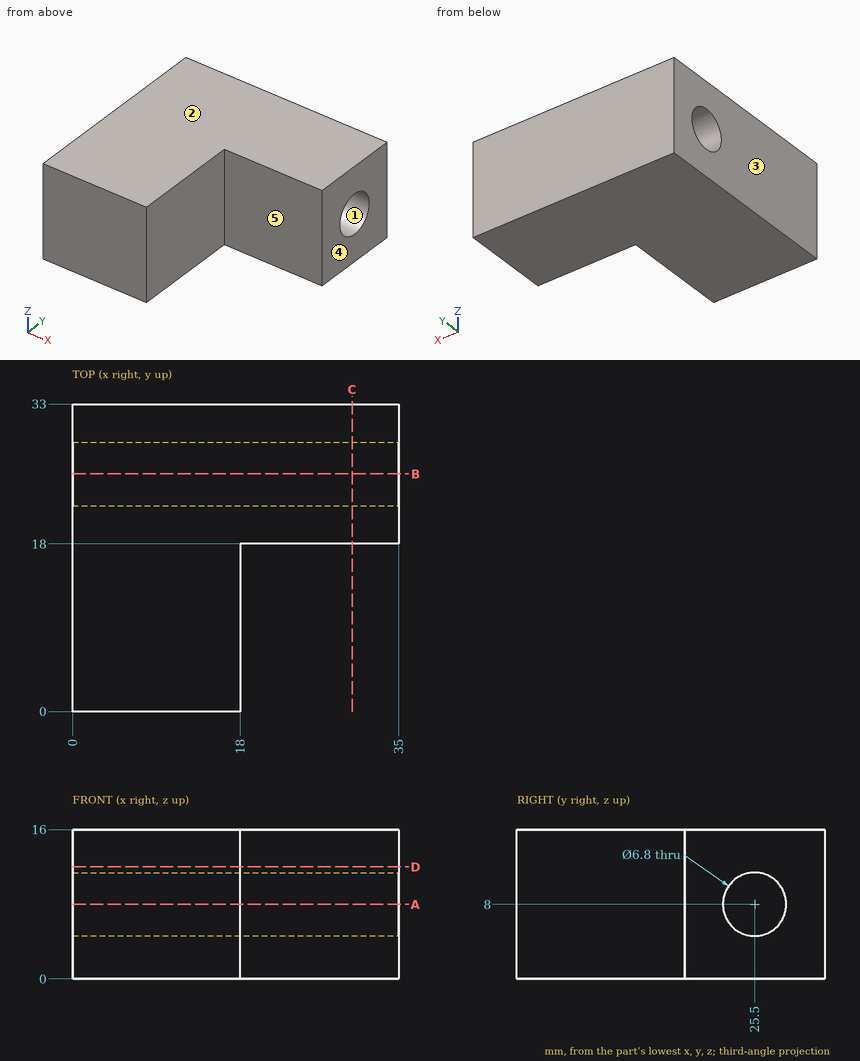
Geometry check sheet. Reference: drawing and pictorial views, mm from the part's lowest x, y, z. A direction names the side the tool comes from. Round coordinates to 2 decimals unless told otherwise and drop trailing zeros. Loops run counter-clockwise (first coordinate to the right, second up) from the corner with the lowest first, then second, coordinate; pieces in that order, holes last. Notation, with made-up numbers: (88, 16) - (127, 16) arc R9 cw to (127, 26) - close; hole circle Ø4 at (45.25, 44). An arc over 180 degrees is marked (long way). Use a Markdown table: item, result. Add a question column.
1. Access from +Z, -Z, +X, -X, +Y, -Y to the whole of each face (thin tool, end or side, straight path). Record for the marked faces 4 and 5.
2. Thickness scan on probe 1 along Y at (x, z) = (19.5, 8); probe 2 along Y at (x, z) = (13, 8); probe 3 along X at (y, z) = (6, 3.5). Record the ranges inside material, lowest first. Write a range as [from, to].
3. Section check B-B, the plane y = 25.5. Record the boundary of the cut face in (x, z), plus the area to 3 significant figures.
4. Gauge pin test, flat end, axial feed: pin 1 (8 mm diameter, centred on x = 28.5, z = 2.5, fed in from -Y). Record the tip position at first contact, or that the pin passes through.
5. Section check C-C, the plane x = 30. Record the boundary of the cut face in (y, z).
6. Release check for a two-part mould opening along Z. For the marked faces 1, 2 and 3 record: released by +Z, released by -Z, zero draft, split by the parting line, or undercut.
7. Section check A-A, the plane z = 8. Record the boundary of the cut face in (x, y), plus the area to 3 significant figures.
8. Section check D-D, the plane z = 12. Record the boundary of the cut face in (x, y), plus the area to 3 significant figures.
Checks:
| question | item | result |
|---|---|---|
| 1 | face 4 | +Z, -Z, +X, +Y, -Y |
| 1 | face 5 | +Z, -Z, +X, -Y |
| 2 | probe 1 | y = [18, 22.1], [28.9, 33] |
| 2 | probe 2 | y = [0, 22.1], [28.9, 33] |
| 2 | probe 3 | x = [0, 18] |
| 3 | outline | (0, 0) - (35, 0) - (35, 4.6) - (0, 4.6) - close; (0, 11.4) - (35, 11.4) - (35, 16) - (0, 16) - close |
| 3 | area | 322 mm^2 |
| 4 | pin 1 | stops at y = 18 |
| 5 | outline | (18, 0) - (33, 0) - (33, 16) - (18, 16) - close; hole circle Ø6.8 at (25.5, 8) |
| 6 | face 1 | undercut |
| 6 | face 2 | released by +Z |
| 6 | face 3 | zero draft |
| 7 | outline | (0, 0) - (18, 0) - (18, 18) - (35, 18) - (35, 22.1) - (0, 22.1) - close; (0, 28.9) - (35, 28.9) - (35, 33) - (0, 33) - close |
| 7 | area | 611 mm^2 |
| 8 | outline | (0, 0) - (18, 0) - (18, 18) - (35, 18) - (35, 33) - (0, 33) - close |
| 8 | area | 849 mm^2 |
